Source: CAD feature listing. Evaluate the final solid. Frame: model axes, mm. Coordinates: 2 decimals unless noted, no trailing zeros. Loops run counter-clockwise (first coordinate to the right, second up) from the corner with the lowest first, then second, coordinate; pieces in that order, holes last. Notation, with made-up numbers: (-9, -12) -> (8, -12) arc R22 cw to (8, 1) -> close; hole circle Ø10 at (-31, 16.25). An arc over 180 degrees is marked (long way). Answer as CSV lines item,"result".
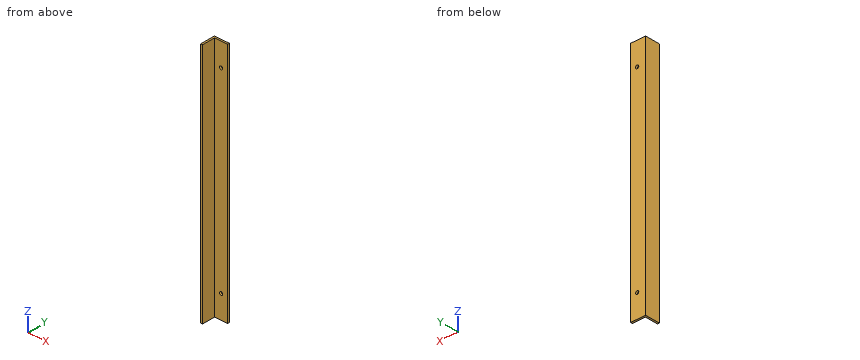
Autodesk Fusion 360 part; units mm, degrees
sketch "Sketch1" plane through (0, 0, 0) normal (0, 0, 1) x (1, 0, 0)
  line L0 (0, 0) -> (25.4, 0)
  line L1 (0, 0) -> (0, -25.4)
  line L2 (3.175, -3.175) -> (25.4, -3.175)
  line L3 (3.175, -3.175) -> (3.175, -25.4)
  line L4 (25.4, 0) -> (25.4, -3.175)
  line L5 (0, -25.4) -> (3.175, -25.4)
  dimension "d1" = 25.4
  dimension "d2" = -3.175
extrude "Extrude1" add sketch "Sketch1" along normal blind 410
sketch "Sketch2" plane through (0, -3.175, 0) normal (0, -1, 0) x (1, 0, 0)
  line L0 (3.175, 0) -> (25.4, 0)
  line L1 (25.4, 0) -> (25.4, 410)
  line L2 (25.4, 410) -> (3.175, 410)
  line L3 (3.175, 410) -> (3.175, 0)
  circle A0 centre (14.2875, 370.71) radius 4.4166
  circle A1 centre (14.2875, 39.29) radius 4.4166
  line L4 (14.2875, 410) -> (14.2875, 0) construction
  line L5 (14.2875, 205) -> (25.4, 205) construction
  dimension "d6" = 165.71
  dimension "d7" = 165.71
hole "Hole1" at (14.2875, -3.175, 370.71) at (14.2875, -3.175, 39.29) direction (0, 1, 0) diameter 5.5 depth 7 tip angle 118
(1) Cut plane B-B (x = 21.5). Return the cut outline in (y, z) (3 decimals).
Computed values:
outline,"(-3.175, 0) -> (0, 0) -> (0, 410) -> (-3.175, 410) -> close"
(2) Material intervals for L1, parallel to X at y = -2.5, z = 370.71; L2, parallel to Z at x = 14, y = -2.5; L3, parallel to Y at x = 16.75, z = 261.5 (3 decimals), sorted ascending. Write a range as [from, to].
Computed values:
L1,"[0, 11.54], [17.04, 25.4]"
L2,"[0, 36.56], [42.02, 367.98], [373.44, 410]"
L3,"[-3.175, 0]"
(3) Pin query (flat end, axial travel): pin 1 Ø5 at (x, z) = (8.5, 261) entering from -Y (3 decimals); pin 2 Ø5 at (y, z) = (-22, 253) entering from +X (3 decimals). Return the tip coordinate at first contact, or that it passes through.
Computed values:
pin 1,"y = -3.175"
pin 2,"x = 3.175"
(4) Cut plane C-C (y = -16.5). Return the cut outline in (x, z) (3 decimals).
Computed values:
outline,"(0, 0) -> (3.175, 0) -> (3.175, 410) -> (0, 410) -> close"
(5) Cut plane A-A (z = 221.5). Return the cut outline in (x, y) (3 decimals), then the cut area to 3 significant figures.
Computed values:
outline,"(0, -25.4) -> (3.175, -25.4) -> (3.175, -3.175) -> (25.4, -3.175) -> (25.4, 0) -> (0, 0) -> close"
area,"151 mm^2"
